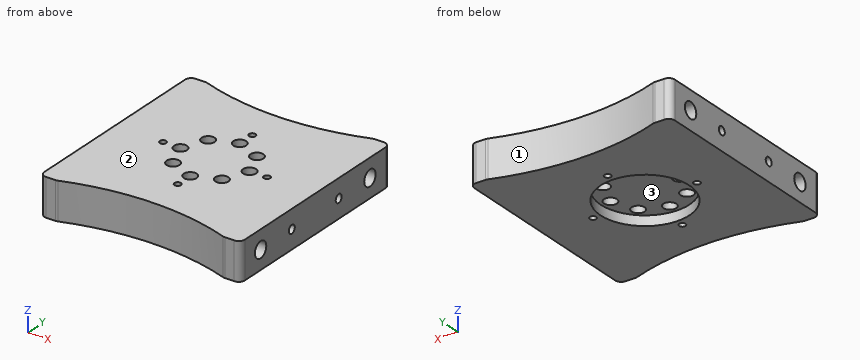
from build123d import *

# Parameters (mm, degrees)
BOSS_EXTRUDE1_DEPTH                         = 19.05
F_1_3_4_CLEARANCE_HOLE1_D                   = 45
F_1_3_4_CLEARANCE_HOLE1_DEPTH               = 5
F_1_4_CLEARANCE_HOLE3_D                     = 6.6
F_1_4_CLEARANCE_HOLE3_DEPTH                 = 19.05
BOSS_EXTRUDE2_DEPTH                         = 19.05
SKETCH21_R                                  = 30
CUT_EXTRUDE1_DEPTH                          = 81.6728269
BOSS_EXTRUDE5_DEPTH                         = 19.05
BOSS_EXTRUDE6_DEPTH                         = 19.05
FILLET2_R                                   = 13
SKETCH29_W                                  = 12.7
SKETCH29_H                                  = 60
BOSS_EXTRUDE7_DEPTH                         = 19.05
BOSS_EXTRUDE8_START                         = -19.05
BOSS_EXTRUDE8_DEPTH                         = 19.05
FILLET3_R                                   = 3.175
F_8_0MM_DOWEL_HOLE1_AT_2_COUNT              = 2
F_8_0MM_DOWEL_HOLE1_AT_2_PITCH              = 77.249249372
TAPPED_HOLE_FOR_M4X0_7_HELICOIL1_AT_2_COUNT = 2
TAPPED_HOLE_FOR_M4X0_7_HELICOIL1_AT_2_PITCH = 33.106821059
F_4_CLEARANCE_HOLE2_D                       = 3.2999934


# Read off the part's stored shape, not the designer's step: Markup2
with BuildPart() as part:
    # Sketch1 → Boss-Extrude1 (new body)
    with BuildSketch(Plane(origin=(0, 0, 0), x_dir=(-1, 0, 0), z_dir=(0, 0, -1))):
        with BuildLine():
            Line((44.45, 0), (44.45, 60))
            Line((44.45, 60), (-44.45, 60))
            Line((-44.45, 60), (-44.45, 0))
            ThreePointArc((-44.45, 0), (0, -44.45), (44.45, 0))
        make_face()
    extrude(amount=-BOSS_EXTRUDE1_DEPTH)

    # 1-3/4 Clearance Hole1
    with Locations(Plane(origin=(0, 0, 0), x_dir=(-1, 0, 0), z_dir=(0, 0, -1))):
        with Locations((-6, 0)):
            Hole(F_1_3_4_CLEARANCE_HOLE1_D / 2, depth=F_1_3_4_CLEARANCE_HOLE1_DEPTH)

    # 1/4 Clearance Hole3
    with Locations(Plane.XY.offset(19.05)):
        with Locations((18.374368671, 12.374368671), (23.499999956, -0.001247108), (18.374368671, -12.374368671), (6, -17.5), (-6.374368671, -12.374368671), (-11.5, 0), (-6.374368671, 12.374368671), (6, 17.5)):
            Hole(F_1_4_CLEARANCE_HOLE3_D / 2, depth=F_1_4_CLEARANCE_HOLE3_DEPTH)

    # Sketch18 → Boss-Extrude2 (add)
    with BuildSketch(Plane(origin=(0, 0, 0), x_dir=(-1, 0, 0), z_dir=(0, 0, -1))):
        with BuildLine():
            Line((-44.45, 0), (-50.45, 0))
            ThreePointArc((-50.45, 0), (-37.430896424, -31.430896424), (-6, -44.45))
            Line((-6, -44.45), (0, -44.45))
            ThreePointArc((0, -44.45), (-31.430896424, -31.430896424), (-44.45, 0))
        make_face()
    extrude(amount=-BOSS_EXTRUDE2_DEPTH)

    # Sketch21 → Cut-Extrude1 (cut, through all)
    with BuildSketch(Plane.XY.offset(19.05)):
        with BuildLine():
            Line((-44.45, 60), (-44.45, 0))
            ThreePointArc((-44.45, 0), (-31.430896424, -31.430896424), (0, -44.45))
            Line((0, -44.45), (6, -44.45))
            ThreePointArc((6, -44.45), (37.430896424, -31.430896424), (50.45, 0))
            Line((50.45, 0), (44.45, 0))
            Line((44.45, 0), (44.45, 60))
            Line((44.45, 60), (-44.45, 60))
        make_face()
        with Locations((5.999999978, -0.000623554)):
            Circle(SKETCH21_R, mode=Mode.SUBTRACT)
    extrude(amount=-CUT_EXTRUDE1_DEPTH, mode=Mode.SUBTRACT)

    # Sketch22 → Boss-Extrude5 (add)
    with BuildSketch(Plane.XY.offset(19.05)):
        with BuildLine():
            Line((44.099999978, -30.000623554), (44.099999978, 29.999376446))
            Line((44.099999978, 29.999376446), (5.999999978, 29.999376446))
            ThreePointArc((5.999999978, 29.999376446), (35.999999978, -0.000623554), (5.999999978, -30.000623554))
            Line((5.999999978, -30.000623554), (44.099999978, -30.000623554))
        make_face()
    boss_extrude5 = extrude(amount=-BOSS_EXTRUDE5_DEPTH)

    # Mirror1: Boss-Extrude5 across plane
    add(boss_extrude5.mirror(Plane(origin=(5.999999978, 0, 0), x_dir=(0, 0, 1), z_dir=(1, 0, 0))))

    # Sketch28 → Boss-Extrude6 (add)
    with BuildSketch(Plane.XY.offset(19.05)):
        with BuildLine():
            Line((-26.798858004, 29.999376446), (38.798858004, 29.999376446))
            ThreePointArc((38.798858004, 29.999376446), (6, 44.448752892), (-26.798858004, 29.999376446))
        make_face()
        with BuildLine():
            ThreePointArc((-26.798858004, -30.000623554), (6, -44.45), (38.798858004, -30.000623554))
            Line((38.798858004, -30.000623554), (-26.798858004, -30.000623554))
        make_face()
    extrude(amount=-BOSS_EXTRUDE6_DEPTH)

    # Fillet2
    fillet2_edges = [part.edges().sort_by_distance(p)[0] for p in [
        (-26.798858004, 29.999376446, 9.525),
        (38.798858004, 29.999376446, 9.525),
        (38.798858004, -30.000623554, 9.525),
        (-26.798858004, -30.000623554, 9.525),
    ]]
    fillet(fillet2_edges, radius=FILLET2_R)

    # Sketch29 → Boss-Extrude7 (add)
    with BuildSketch(Plane.XY):
        with Locations((50.449999978, -0.000623554)):
            Rectangle(SKETCH29_W, SKETCH29_H)
        with Locations((-38.447885426, -0.000623554)):
            Rectangle(SKETCH29_W, SKETCH29_H)
    extrude(amount=BOSS_EXTRUDE7_DEPTH)

    # Sketch40 → Boss-Extrude8 (add)
    with BuildSketch(Plane.XY.offset(19.05).offset(BOSS_EXTRUDE8_START)):
        with BuildLine():
            Line((56.799999978, -30.000623554), (44.097885426, -30.000623554))
            ThreePointArc((44.097885426, -30.000623554), (39.487811488, -30.845492198), (35.476953998, -33.27028228))
            ThreePointArc((35.476953998, -33.27028228), (6, -44.45), (-23.476953998, -33.27028228))
            ThreePointArc((-23.476953998, -33.27028228), (-27.487811488, -30.845492198), (-32.097885426, -30.000623554))
            Line((-32.097885426, -30.000623554), (-44.797885426, -30.000623554))
            Line((-44.797885426, -30.000623554), (-44.797885426, -52.835855224))
            Line((-44.797885426, -52.835855224), (-36.33121876, -52.835855224))
            ThreePointArc((-36.33121876, -52.835855224), (6.001057276, -45.572977311), (48.333333311, -52.835855224))
            Line((48.333333311, -52.835855224), (56.799999978, -52.835855224))
            Line((56.799999978, -52.835855224), (56.799999978, -30.000623554))
        make_face()
        with BuildLine():
            Line((-36.33121876, 52.834608116), (-44.797885426, 52.834608116))
            Line((-44.797885426, 52.834608116), (-44.797885426, 29.999376446))
            Line((-44.797885426, 29.999376446), (-32.097885426, 29.999376446))
            ThreePointArc((-32.097885426, 29.999376446), (-27.487811488, 30.84424509), (-23.476953998, 33.269035172))
            ThreePointArc((-23.476953998, 33.269035172), (6, 44.448752892), (35.476953998, 33.269035172))
            ThreePointArc((35.476953998, 33.269035172), (39.487811488, 30.84424509), (44.097885426, 29.999376446))
            Line((44.097885426, 29.999376446), (56.799999978, 29.999376446))
            Line((56.799999978, 29.999376446), (56.799999978, 52.834608116))
            Line((56.799999978, 52.834608116), (48.333333311, 52.834608116))
            ThreePointArc((48.333333311, 52.834608116), (6.001057276, 45.571730203), (-36.33121876, 52.834608116))
        make_face()
    extrude(amount=BOSS_EXTRUDE8_DEPTH)

    # Fillet3
    fillet3_edges = [part.edges().sort_by_distance(p)[0] for p in [
        (-44.797885426, -52.835855224, 9.525),
        (-36.33121876, -52.835855224, 9.525),
        (48.333333311, -52.835855224, 9.525),
        (56.799999978, -52.835855224, 9.525),
        (56.799999978, 52.834608116, 9.525),
        (48.333333311, 52.834608116, 9.525),
        (-36.33121876, 52.834608116, 9.525),
        (-44.797885426, 52.834608116, 9.525),
    ]]
    fillet(fillet3_edges, radius=FILLET3_R)

    # Sketch49 → Ø8.0mm Dowel Hole1 (revolve, cut)
    with BuildSketch(Plane(origin=(56.799999978, 38.624001078, 9.525), x_dir=(0, 0, -1), z_dir=(0, 1, 0))):
        Polygon((0, 0), (0, 27.818463992), (4.025, 25.4), (4.025, 0), align=None)
    f_8_0mm_dowel_hole1 = revolve(axis=Axis((63.149999978, 38.624001078, 9.525), (-1, 0, 0)), mode=Mode.SUBTRACT)

    # Ø8.0mm Dowel Hole1 at 2: Ø8.0mm Dowel Hole1 ×2
    with Locations(*[(0, -i * F_8_0MM_DOWEL_HOLE1_AT_2_PITCH, 0) for i in range(1, F_8_0MM_DOWEL_HOLE1_AT_2_COUNT)]):
        add(f_8_0mm_dowel_hole1, mode=Mode.SUBTRACT)

    # Sketch52 → Tapped Hole for M4x0.7 Helicoil1 (revolve, cut)
    with BuildSketch(Plane(origin=(56.799999978, 16.552787003, 9.525), x_dir=(0, 0, -1), z_dir=(0, 1, 0))):
        Polygon((0, 0), (0, 13.4538073), (2.1, 12.192), (2.1, 0), align=None)
    tapped_hole_for_m4x0_7_helicoil1 = revolve(axis=Axis((63.149999978, 16.552787003, 9.525), (-1, 0, 0)), mode=Mode.SUBTRACT)

    # Tapped Hole for M4x0.7 Helicoil1 at 2: Tapped Hole for M4x0.7 Helicoil1 ×2
    with Locations(*[(0, -i * TAPPED_HOLE_FOR_M4X0_7_HELICOIL1_AT_2_PITCH, 0) for i in range(1, TAPPED_HOLE_FOR_M4X0_7_HELICOIL1_AT_2_COUNT)]):
        add(tapped_hole_for_m4x0_7_helicoil1, mode=Mode.SUBTRACT)

    # Mirror6: Ø8.0mm Dowel Hole1, Tapped Hole for M4x0.7 Helicoil1 across plane
    add(f_8_0mm_dowel_hole1.mirror(Plane(origin=(5.999999978, 0, 0), x_dir=(0, 0, 1), z_dir=(1, 0, 0))), mode=Mode.SUBTRACT)
    add(tapped_hole_for_m4x0_7_helicoil1.mirror(Plane(origin=(5.999999978, 0, 0), x_dir=(0, 0, 1), z_dir=(1, 0, 0))), mode=Mode.SUBTRACT)

    # Mirror6 copy 1 sketch → Mirror6 copy 1 (revolve, cut)
    with BuildSketch(Plane(origin=(-44.800000022, -38.625248294, 9.525), x_dir=(0, 0, -1), z_dir=(0, 1, 0))):
        Polygon((0, 0), (0, -27.818463992), (4.025, -25.4), (4.025, 0), align=None)
    revolve(axis=Axis((-51.150000022, -38.625248294, 9.525), (-1, 0, 0)), mode=Mode.SUBTRACT)

    # Mirror6 copy 2 sketch → Mirror6 copy 2 (revolve, cut)
    with BuildSketch(Plane(origin=(-44.800000022, -16.554034056, 9.525), x_dir=(0, 0, -1), z_dir=(0, 1, 0))):
        Polygon((0, 0), (0, -13.4538073), (2.1, -12.192), (2.1, 0), align=None)
    revolve(axis=Axis((-51.150000022, -16.554034056, 9.525), (-1, 0, 0)), mode=Mode.SUBTRACT)

    # #4 Clearance Hole2 (through all)
    with Locations(Plane.XY.offset(19.05)):
        with Locations((32.350000005, 0), (6, 26.350000005), (-20.350000005, 0), (6, -26.350000005)):
            Hole(F_4_CLEARANCE_HOLE2_D / 2)


solid = part.part
Check sheet for the modelled part. Datum: model origin and axes. Units: mm. Face numbers are marked on the shaded views. Give positions to 0.01 mm unless a question says otherwise; leave off trailing zeros. Write each loop counter-clockwise with the first axis right and the second up, starting at its lowest first coordinate (ties: lowest second). Pieces come first, ordered by that corner, then holes. Notation, with made-up numbers: M 80,69.5 L 139,69.5 A32 ccw 139,98.5 Z; hole C 88.5,-8 d11. An arc over 180 degrees is marked long. Use one line per item in the form item = value.
(1) Section check D-D on z = 17.75. State how many separate pieces and enclosed holes the cut face has, plus the area to 3 significant figures.
Answer block:
separate_pieces = 1
enclosed_holes = 12
area = 9,590 mm2
(2) Material ranges on line 1 along Y through (x, z) = (47.5, 10.5); line 2 along Y through (x, z) = (-32, 13); line 3 along Z through (x, y) = (-4, -19.5), recorded low to high.
Answer block:
line_1 = -52.54 to -42.53, -34.72 to -18.41, -14.69 to 14.69, 18.41 to 34.72, 42.53 to 52.54
line_2 = -51.39 to -40.66, -36.59 to 36.59, 40.66 to 51.39
line_3 = 5 to 19.05
(3) Section check A-A on y = 26.35. Record the boundary of the cut face in (x, z).
Answer block:
outline = M -44.8,0 L 4.35,0 L 4.35,19.05 L -44.8,19.05 Z; M 7.65,0 L 56.8,0 L 56.8,19.05 L 7.65,19.05 Z
(4) Section check B-B on z = 3. Record the boundary of the cut face in (x, y) (3 decimals), plus the area to 3 significant figures.
Answer block:
outline = M -44.798,-49.661 A3.175 ccw -41.623,-52.836 L -36.872,-52.836 A3.175 ccw -35.827,-52.659 A127 cw 47.829,-52.659 A3.175 ccw 48.875,-52.836 L 53.625,-52.836 A3.175 ccw 56.8,-49.661 L 56.8,49.66 A3.175 ccw 53.625,52.835 L 48.875,52.835 A3.175 ccw 47.829,52.657 A127 cw -35.827,52.657 A3.175 ccw -36.872,52.835 L -41.623,52.835 A3.175 ccw -44.798,49.66 Z; hole C -20.35,0 d3.3; hole C 6,0 d45; hole C 6,-26.35 d3.3; hole C 6,26.35 d3.3; hole C 32.35,0 d3.3
area = 8,280 mm2
(5) Draft check along Y on the marked faces 1, 2 and 3. Enter one of: pulls with the +Y half, pulls with the -Y half, needs draft (parallel to the pull), parting line crosses it, or undercut.
Answer block:
face_1 = pulls with the +Y half
face_2 = needs draft
face_3 = undercut
(6) Depth check by flat-ended pin: P1, Ø2.5, axis at x = 6, y = 26.35, coming from the -Z side; P2, Ø3.5, axis at y = -16.55, z = 9.52, coming from the -X side; P3, Ø4, axis at x = -8, z = 13.5, coming from the -Y side (3 decimals); P4, Ø13.5, axis at x = -3, y = -0.5, coming from the -Z side. Enter the tip coordinate at first touch or a pass-through.
Answer block:
P1 = through
P2 = -32.4
P3 = -46.585
P4 = 5
(7) Section check C-C on x = 46.5. Record the boundary of the cut face in (y, z) (3 decimals), plus the area to 3 significant figures.
Answer block:
outline = M -52.203,0 L 52.202,0 L 52.202,19.05 L -52.203,19.05 Z; hole C -38.625,9.525 d8.05; hole C -16.554,9.525 d4.2; hole C 16.553,9.525 d4.2; hole C 38.624,9.525 d8.05
area = 1,860 mm2
